Part model, mm, in its own coordinate system. Face numbers are marked on the shaded views. A direction names the side the tool comes from. Round coordinates to 2 decimals unless told otherwise and drop trailing zeros. Write each loop counter-clockwise with the first axis right and the second up, starting at its lowest first coordinate (ties: lowest second). Pieces come first, ordered by that corner, then holes.
1) Saw through at B-B on z = 21. Write the cut outline in (x, y).
2) Which spindle directions (+Z, -Z, +X, -X, +Y, -Y) get a long thin tool onto all of the face, cutting with end or side? Do the marked faces 1, 2 and 3. Say none if no direction does.
3) Saw through at C-C on x = 0. Write the cut outline in (y, z), and give its area (3 significant figures).
4) Saw through at A-A on z = 30. Write the cut outline in (x, y).
5) Saw through at D-D on y = 3.25. Count the separate pieces of the cut face and the enclosed holes in it, and give its area (3 significant figures).
6) Flat gauge pins, fed straight in: pin 1 (9 mm diameter, centred on x = 28.12, z = 10, fed in from +Y); pin 2 (4 mm diameter, centred on y = 15.5, z = 28.5, fed in from -X); pin 3 (7.5 mm diameter, centred on x = -30, z = 19, fed in from +Y). Where does each tip first touch, or does it go through?
7) Drill centre lines: L1, parallel to X at y = 0.5, z = 30; L2, parallel to X at y = 2.5, z = 27; L3, parallel to Y at x = -27.5, z = 33. Where is each one in solid material? Low to high.
```python
from build123d import *

# Parameters (mm, degrees)
ESTRUSIONE_ESTRUSIONE1_DEPTH                         = 40
FORO_LAMATO_PER_VITE_M4_A_TESTA_CILINDRI_D           = 4.5
FORO_LAMATO_PER_VITE_M4_A_TESTA_CILINDRI_DEPTH       = 80
FORO_LAMATO_PER_VITE_M4_A_TESTA_CILINDRI_CBORE_D     = 10
FORO_LAMATO_PER_VITE_M4_A_TESTA_CILINDRI_CBORE_DEPTH = 2.6
FORO_LAMATO_PER_VITE_M4_A_TESTA_CILINDRI_TIP         = 1.351936393
SMUSSO1_SIZE                                         = 2
TAGLIO_ESTRUSIONE1_DEPTH                             = 10


with BuildPart() as part:
    # Schizzo1 → Estrusione-Estrusione1 (new body)
    with BuildSketch(Plane.XY):
        with BuildLine():
            Line((-15, 0), (-38.615528128, 0))
            Line((-38.615528128, 0), (-35.615528128, 4))
            Line((-35.615528128, 4), (-20.615528128, 4))
            ThreePointArc((-20.615528128, 4), (0, 21), (20.615528128, 4))
            Line((20.615528128, 4), (35.615528128, 4))
            Line((35.615528128, 4), (38.615528128, 0))
            Line((38.615528128, 0), (15, 0))
            ThreePointArc((15, 0), (0, 15), (-15, 0))
        make_face()
    extrude(amount=ESTRUSIONE_ESTRUSIONE1_DEPTH)

    # Foro lamato per Vite M4 a testa cilindrica-1
    with Locations(Plane(origin=(0, 4, 0), x_dir=(1, 0, 0), z_dir=(0, 1, 0))):
        with Locations((-28.115528128, -10), (-28.115528128, -30), (28.115528128, -30), (28.115528128, -10)):
            CounterBoreHole(FORO_LAMATO_PER_VITE_M4_A_TESTA_CILINDRI_D / 2, FORO_LAMATO_PER_VITE_M4_A_TESTA_CILINDRI_CBORE_D / 2, FORO_LAMATO_PER_VITE_M4_A_TESTA_CILINDRI_CBORE_DEPTH, depth=FORO_LAMATO_PER_VITE_M4_A_TESTA_CILINDRI_DEPTH)
            with Locations((0, 0, -(FORO_LAMATO_PER_VITE_M4_A_TESTA_CILINDRI_DEPTH + FORO_LAMATO_PER_VITE_M4_A_TESTA_CILINDRI_TIP / 2))):  # 118° drill point
                Cone(0, FORO_LAMATO_PER_VITE_M4_A_TESTA_CILINDRI_D / 2, FORO_LAMATO_PER_VITE_M4_A_TESTA_CILINDRI_TIP, mode=Mode.SUBTRACT)

    # Smusso1
    smusso1_edges = [part.edges().sort_by_distance(p)[0] for p in [
        (28.115528128, 4, 0),
        (28.115528128, 4, 40),
        (0, 21, 40),
        (-28.115528128, 4, 40),
        (-28.115528128, 4, 0),
        (0, 21, 0),
    ]]
    chamfer(smusso1_edges, length=SMUSSO1_SIZE)

    # Schizzo4 → Taglio-Estrusione1 (cut)
    with BuildSketch(Plane.XZ):
        Polygon((-38.615528128, 38), (-36.615528128, 40), (-38.615528128, 40), align=None)
        Polygon((-38.615528128, 2), (-36.615528128, 0), (-38.615528128, 0), align=None)
        Polygon((36.615528128, 0), (38.615528128, 2), (38.615528128, 0), align=None)
        Polygon((36.615528128, 40), (38.615528128, 40), (38.615528128, 38), align=None)
    extrude(amount=-TAGLIO_ESTRUSIONE1_DEPTH, mode=Mode.SUBTRACT)


solid = part.part
```
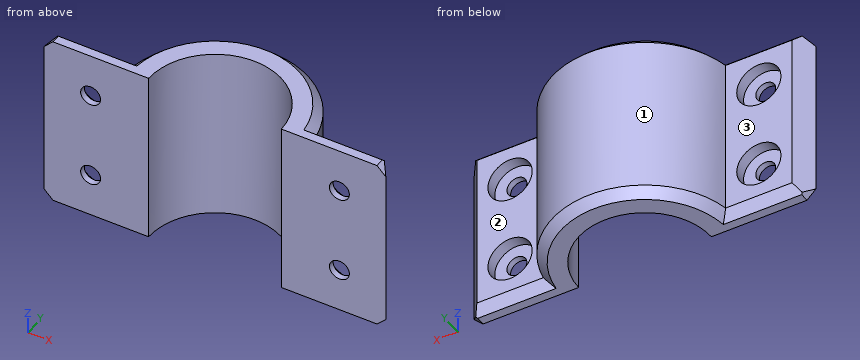
Completed:
1. outline: (-38.62, 0) - (-15, 0) arc R15 cw to (15, 0) - (38.62, 0) - (35.62, 4) - (20.62, 4) arc R21 ccw to (-20.62, 4) - (-35.62, 4) - close
2. face 1: +Z, -Z, +Y
2. face 2: +Z, -Z, +X, +Y
2. face 3: +Z, -Z, -X, +Y
3. outline: (15, 0) - (19, 0) - (21, 2) - (21, 38) - (19, 40) - (15, 40) - close
3. area: 236 mm2
4. outline: (-38.62, 0) - (-30.37, 0) - (-30.37, 1.4) - (-33.12, 1.4) - (-33.12, 4) - (-35.62, 4) - close; (-25.87, 0) - (-15, 0) arc R15 cw to (15, 0) - (25.87, 0) - (25.87, 1.4) - (23.12, 1.4) - (23.12, 4) - (20.62, 4) arc R21 ccw to (-20.62, 4) - (-23.12, 4) - (-23.12, 1.4) - (-25.87, 1.4) - close; (30.37, 0) - (38.62, 0) - (35.62, 4) - (33.12, 4) - (33.12, 1.4) - (30.37, 1.4) - close
5. separate pieces: 2
5. enclosed holes: 4
5. area: 1,320 mm2
6. pin 1: stops at y = 1.4
6. pin 2: stops at x = -16.09
6. pin 3: stops at y = 4
7. L1: x = -38.24 to -30.37, -25.87 to -14.99, 14.99 to 25.87, 30.37 to 38.24
7. L2: x = -36.74 to -32.12, -24.12 to -14.79, 14.79 to 24.12, 32.12 to 36.74
7. L3: y = 0 to 1.4
